```python
from build123d import *

# Parameters (mm, degrees)
SKETCH1_W           = 70
SKETCH1_H           = 50
BOSS_EXTRUDE1_DEPTH = 10
BOSS_EXTRUDE2_DEPTH = 40
BOSS_EXTRUDE3_DEPTH = 50


with BuildPart() as part:
    # Sketch1 → Boss-Extrude1 (new body)
    with BuildSketch(Plane(origin=(0, 0, 0), x_dir=(1, 0, 0), z_dir=(0, 1, 0))):
        Rectangle(SKETCH1_W, SKETCH1_H)
    extrude(amount=BOSS_EXTRUDE1_DEPTH)

    # Sketch3 → Boss-Extrude2 (add)
    with BuildSketch(Plane(origin=(0, 10, 0), x_dir=(1, 0, 0), z_dir=(0, 1, 0))):
        Polygon((-35, 25), (0, 25), (0, 0), (-15, 0), (-15, -25), (-35, -25), align=None)
    extrude(amount=BOSS_EXTRUDE2_DEPTH)

    # Sketch4 → Boss-Extrude3 (add)
    with BuildSketch(Plane(origin=(35, 0, 0), x_dir=(0, 0, -1), z_dir=(1, 0, 0))):
        Polygon((25, 10), (25, 28), (0, 50), (-25, 10), align=None)
    extrude(amount=-BOSS_EXTRUDE3_DEPTH)


solid = part.part
```
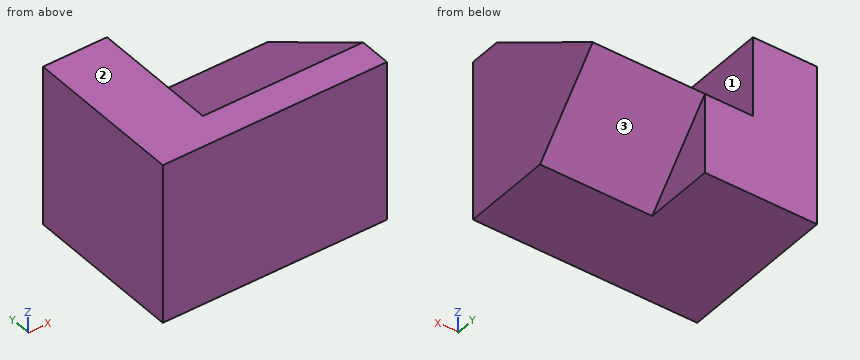
Input: part model. Units: mm. Frame: model coordinates. Face numbers are marked on the shaded views. A direction names the side the tool comes from. Coordinates: 2 decimals unless noted, no trailing zeros. Loops run counter-clockwise (first coordinate to the right, second up) from the corner with the lowest first, then second, coordinate; pieces in that order, holes last.
Q1. Section D-D, the plane z = 2.5. Return the cut outline in (x, y).
Results are:
outline: (-35, 0) - (35, 0) - (35, 46) - (-15, 46) - (-15, 50) - (-35, 50) - close
Q2. Section A-A, the plane x = -12.5. Return the cut outline in (y, z).
Results are:
outline: (0, -25) - (50, -25) - (50, 0) - (10, 25) - (0, 25) - close
Q3. Section C-C, the plane y = 44.5. Return the cut outline in (x, z), and give its area (3 significant figures).
Results are:
outline: (-35, -25) - (0, -25) - (0, -6.25) - (35, -6.25) - (35, 3.44) - (-15, 3.44) - (-15, 25) - (-35, 25) - close
area: 1,770 mm2
Q4. Section B-B, the plane z = 8. Return the cut outline in (x, y), and give its area (3 significant figures).
Results are:
outline: (-35, 0) - (35, 0) - (35, 37.2) - (-15, 37.2) - (-15, 50) - (-35, 50) - close
area: 2,860 mm2
Q5. Set-up query: the marked faces 1, 2 and 3. Return all of +Z, -Z, +X, -X, +Y, -Y with unobstructed straight access to the full face (end or side cutting, diameter ignored); none if empty.
Results are:
face 1: +Z, +X, +Y
face 2: +Z, +X, -X, +Y, -Y
face 3: -Z, +X, +Y
Q6. Line query: line 1 along X through (y, z) = (39.5, -16); line 2 along X through (y, z) = (40, 15); line 3 along Y through (x, z) = (28.5, -22.5). Output: solid intervals per line, ascending.
Results are:
line 1: x = -35 to 0
line 2: x = -35 to -15
line 3: y = 0 to 30.2
Q7. Contact query for a flat-ended pin moving along its axis: pin 1 (4 mm diameter, centred on x = -12, y = 42, fed in from +Z). Output: stop coordinate, or through.
Results are:
pin 1: stops at z = 6.25
